Can you work these out from the model? Positions are in its coordinate system, mm. A direction names the side the tool comes from. Round coordinates to 2 decimals unless told otherwise and drop trailing zeros. Order: outer loops, then holes, each group sorted by start corner. A loop starts at its lowest first (then second) coordinate and runs counter-clockwise, first axis right, second up. Notation, with made-up numbers: M 88,-26.5 L 99,-26.5 A31 cw 99,0.5 Z; hole C 72.5,65.5 d1. An arc over 180 degrees is marked long. Answer as a JSON object with one key per item and string values. Group by question number.
from build123d import *

# Parameters (mm, degrees)
BOSS_EXTRUDE1_DEPTH = 3.175
SKETCH2_R           = 2.1828125
CUT_EXTRUDE2_DEPTH  = 47.003133364


with BuildPart() as part:
    # Sketch1 → Boss-Extrude1 (new body)
    with BuildSketch(Plane.XY):
        Polygon((-6.35, -19.05), (-19.05, -19.05), (0, -41.752905939), (19.05, -19.05), (6.35, -19.05), (6.35, 19.05), (-6.35, 19.05), align=None)
    extrude(amount=BOSS_EXTRUDE1_DEPTH)

    # Sketch2 → Cut-Extrude2 (cut, through all)
    with BuildSketch(Plane.XY.offset(3.175)):
        with Locations((0, 14.2875)):
            Circle(SKETCH2_R)
        with Locations(Location((0, 4.7625, 0), (0, 0, 180))):
            Circle(SKETCH2_R)
    extrude(amount=-CUT_EXTRUDE2_DEPTH, mode=Mode.SUBTRACT)


solid = part.part
Item 1: Suppose I cut it at D-D, the plane x = 10. Write out the boundary of the cut face in (y, z) (3 decimals).
Item 2: Suppose I cut it at B-B, the plane x = 1. Write out the boundary of the cut face in (y, z) (3 decimals).
Item 3: I'm going to push flat-ended pins straight in: pin 1 Ø1 at (y, z) = (-22.5, 2) entering from +X; pin 2 Ø5 at (x, y) = (-10.5, -16.5) entering from +Z; pin 3 Ø1.6 at (x, z) = (-13.5, 2) entering from +Y; pin 4 Ø1 at (y, z) = (-1, 2) entering from -X. Where does each tip first touch, or does it pass through?
Item 4: On a 3-axis mill with a long thin cutter (end or side, diameter ignored), from which of +Z, -Z, +X, -X, +Y, -Y can I reach the whole of each face in a straight line? I mean faces 1 (the face through (-13, -19.05, 2)), 2 (the face through (-9.66, -30.24, 1.57)), 3 (the face through (13, -19.05, 2)). Say none if no direction works.
Item 5: Suppose I cut it at C-C, the plane y = -13.5. Write out the boundary of the cut face in (x, z) (3 decimals), and give its area (3 significant figures).
Item 6: If we mould it in two halves opening along X, with no side actions, what happens to faces 4 (the face through (0, -11, 3.175)), 5 (the face through (-6.35, 0, 2)), 6 (the face through (6.35, 0, 2)), 7 (the face through (0.3, 2.6, 1.6))? For each: +X half, -X half, draft (parallel to the pull), parting line (faces both ways), or undercut.
Item 7: I need wall thicknesses on line 1 (X direction, y = -9.5, z = 0.3); line 2 (Y direction, x = 1, z = 2.9); line 3 (X direction, y = 3.5, z = 0.2). Which ranges of each line are inside material? Lowest first, please.
Item 8: Suppose I cut it at A-A, the plane z = 2.1. Write out the boundary of the cut face in (x, y), and give its area (3 significant figures).
Computed:
{
 "1": {"outline": "M -29.835,0 L -19.05,0 L -19.05,3.175 L -29.835,3.175 Z"},
 "2": {"outline": "M -40.561,0 L 2.822,0 L 2.822,3.175 L -40.561,3.175 Z; M 6.703,0 L 12.347,0 L 12.347,3.175 L 6.703,3.175 Z; M 16.228,0 L 19.05,0 L 19.05,3.175 L 16.228,3.175 Z"},
 "3": {"pin 1": "stops at x = 16.57", "pin 2": "passes through", "pin 3": "stops at y = -19.05", "pin 4": "stops at x = -6.35"},
 "4": {"face 1": "+Z, -Z, -X, +Y", "face 2": "+Z, -Z, -X, -Y", "face 3": "+Z, -Z, +X, +Y"},
 "5": {"outline": "M -6.35,0 L 6.35,0 L 6.35,3.175 L -6.35,3.175 Z", "area": "40.3 mm^2"},
 "6": {"face 4": "draft", "face 5": "-X half", "face 6": "+X half", "face 7": "undercut"},
 "7": {"line 1": "x = -6.35 to 6.35", "line 2": "y = -40.56 to 2.82, 6.7 to 12.35, 16.23 to 19.05", "line 3": "x = -6.35 to -1.78, 1.78 to 6.35"},
 "8": {"outline": "M -19.05,-19.05 L 0,-41.75 L 19.05,-19.05 L 6.35,-19.05 L 6.35,19.05 L -6.35,19.05 L -6.35,-19.05 Z; hole C 0,4.76 d4.37; hole C 0,14.29 d4.37", "area": "886 mm^2"}
}
